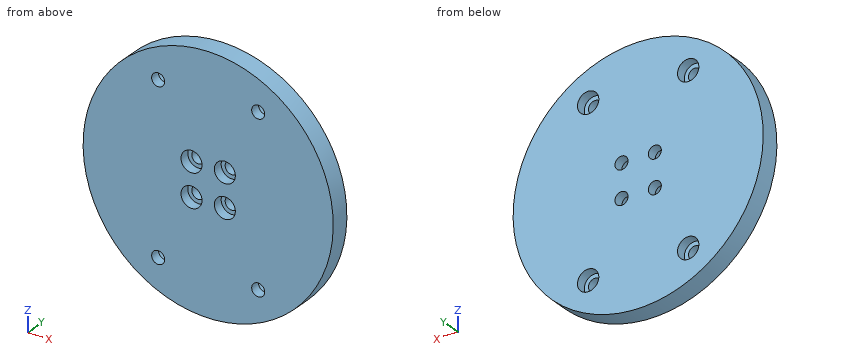
from build123d import *

# Parameters (mm, degrees)
SKIZZE1_R                       = 37.5
AUFSATZ_LINEAR_AUSTRAGEN1_DEPTH = 6
BOHRUNG3_D                      = 3.9
BOHRUNG3_CBORE_D                = 6.3
BOHRUNG3_CBORE_DEPTH            = 3
BOHRUNG4_D                      = 3.9
BOHRUNG4_CBORE_D                = 6.4
BOHRUNG4_CBORE_DEPTH            = 3


with BuildPart() as part:
    # Skizze1 → Aufsatz-Linear austragen1 (new body)
    with BuildSketch(Plane(origin=(0, 0, 0), x_dir=(1, 0, 0), z_dir=(0, 1, 0))):
        with Locations(Location((25, 30, 0), (0, 0, 270))):
            Circle(SKIZZE1_R)
    extrude(amount=AUFSATZ_LINEAR_AUSTRAGEN1_DEPTH)

    # Bohrung3 (through all)
    with Locations(Plane(origin=(20, 0, -25), x_dir=(0, 0, -1), z_dir=(0, -1, 0))):
        with Locations((0, 0), (0, 10), (10, 10), (10, 0)):
            CounterBoreHole(BOHRUNG3_D / 2, BOHRUNG3_CBORE_D / 2, BOHRUNG3_CBORE_DEPTH)

    # Bohrung4 (through all)
    with Locations(Plane(origin=(10, 6, -55), x_dir=(0, 0, 1), z_dir=(0, 1, 0))):
        with Locations((0, 0), (50, 30), (50, 0), (0, 30)):
            CounterBoreHole(BOHRUNG4_D / 2, BOHRUNG4_CBORE_D / 2, BOHRUNG4_CBORE_DEPTH)


solid = part.part
Verification items for the finished model (mm, model axes). Round coordinates to 2 decimals unless told otherwise and drop trailing zeros. Order: outer loops, then holes, each group sorted by start corner. A loop starts at its lowest first (then second) coordinate and runs counter-clockwise, first axis right, second up.
1. Section check C-C on x = 40. Record the cut outline in (y, z).
Final values:
outline: (0, -64.37) - (6, -64.37) - (6, -58.2) - (3, -58.2) - (3, -56.95) - (0, -56.95) - close; (0, -53.05) - (3, -53.05) - (3, -51.8) - (6, -51.8) - (6, -8.2) - (3, -8.2) - (3, -6.95) - (0, -6.95) - close; (0, -3.05) - (3, -3.05) - (3, -1.8) - (6, -1.8) - (6, 4.37) - (0, 4.37) - close
2. Section check B-B on z = -35. Record the cut outline in (x, y), then the cut area to 3 significant figures.
Final values:
outline: (-12.17, 0) - (16.85, 0) - (16.85, 3) - (18.05, 3) - (18.05, 6) - (-12.17, 6) - close; (21.95, 3) - (23.15, 3) - (23.15, 0) - (26.85, 0) - (26.85, 3) - (28.05, 3) - (28.05, 6) - (21.95, 6) - close; (31.95, 3) - (33.15, 3) - (33.15, 0) - (62.17, 0) - (62.17, 6) - (31.95, 6) - close
area: 385 mm2
3. Section check D-D on x = -7.5. Record the cut outline in (y, z).
Final values:
outline: (0, -48.71) - (6, -48.71) - (6, -11.29) - (0, -11.29) - close
4. Go/stop test with flat-tipped pins: P1, Ø2.5, axis at x = 20, z = -25, coming from the +Y side; P2, Ø4.5, axis at x = 10, z = -5, coming from the +Y side; P3, Ø5, axis at x = 20, z = -35, coming from the -Y side; P4, Ø1, axis at y = 1, z = -56, coming from the -X side. Record where each tip stops, or that it passes through.
Final values:
P1: passes through
P2: stops at y = 3
P3: stops at y = 3
P4: stops at x = -2.5
5. Section check A-A on y = 0.9. State how many separate pieces and enclosed holes the cut face has, then the cut area to 3 significant figures.
Final values:
separate pieces: 1
enclosed holes: 8
area: 4,250 mm2
6. Thickness scan on L1, parallel to X at y = 1.3, z = -6; L2, parallel to X at y = 3.8, z = -25; L3, parallel to Z at x = 29.5, y = 0.3. Record the ranges inside material, lowest first.
Final values:
L1: x = -3.81 to 8.33, 11.67 to 38.33, 41.67 to 53.81
L2: x = -12.17 to 18.05, 21.95 to 28.05, 31.95 to 62.17
L3: z = -67.23 to -38.11, -31.89 to -28.11, -21.89 to 7.23
